Part model, mm, in its own coordinate system. A direction names the side the tool comes from. Round coordinates to 2 decimals unless told otherwise and drop trailing zeros. Write each loop counter-clockwise with the first axis right and the second up, starting at its lowest first coordinate (ties: lowest second). Pieces come first, ordered by that corner, then holes.
```python
from build123d import *

# Parameters (mm, degrees)
SKETCH_1_R          = 2.25
EXTRUDE_2_DEPTH     = 20
SKETCH_7_W          = 2.4
SKETCH_7_H          = 2.4
CUT_EXTRUDE_3_DEPTH = 2.5
SKETCH_9_R          = 3
EXTRUDE_4_DEPTH     = 1
SKETCH_10_W         = 4
SKETCH_10_H         = 4
EXTRUDE_5_DEPTH     = 2
CUT_EXTRUDE_START   = -20
SKETCH_12_OUTSIDE_W = 12.904
SKETCH_12_OUTSIDE_H = 12.904
SKETCH_12_OUTSIDE_R = 1
CUT_EXTRUDE_4_DEPTH = 16.5
FILLET_1_R          = 2


with BuildPart() as part:
    # 草图1 → 凸台-拉伸2 (new body)
    with BuildSketch(Plane.XY):
        Circle(SKETCH_1_R)
    extrude(amount=EXTRUDE_2_DEPTH)

    # 草图7 → 切除-拉伸3 (cut)
    with BuildSketch(Plane.XY):
        Rectangle(SKETCH_7_W, SKETCH_7_H)
    extrude(amount=CUT_EXTRUDE_3_DEPTH, mode=Mode.SUBTRACT)

    # 草图9 → 凸台-拉伸4 (add)
    with BuildSketch(Plane.XY.offset(20)):
        Circle(SKETCH_9_R)
    extrude(amount=EXTRUDE_4_DEPTH)

    # 草图10 → 凸台-拉伸5 (add)
    with BuildSketch(Plane.XY.offset(21)):
        Rectangle(SKETCH_10_W, SKETCH_10_H)
    extrude(amount=EXTRUDE_5_DEPTH)

    # 草图12 outside → 切除-拉伸4 (cut)
    with BuildSketch(Plane(origin=(0, 0, 0), x_dir=(-1, 0, 0), z_dir=(0, 0, -1)).offset(CUT_EXTRUDE_START)):
        Rectangle(SKETCH_12_OUTSIDE_W, SKETCH_12_OUTSIDE_H)
        with Locations(Location((0, 0, 0), (0, 0, 180))):
            Circle(SKETCH_12_OUTSIDE_R, mode=Mode.SUBTRACT)
    extrude(amount=CUT_EXTRUDE_4_DEPTH, mode=Mode.SUBTRACT)

    # 圆角1
    # the kernel refuses this fillet: 2 mm, written as the material it adds along each edge
    with BuildSketch(Plane(origin=(0, 0, 3.5), x_dir=(1, 0, 0), z_dir=(0, 1, 0))) as fillet_1_piece_1:
        with BuildLine():
            CenterArc((3, -1.854049622), FILLET_1_R, 112.024312837, 67.975687163)
            Line((2.25, 0), (2.235, 0.037080992))
            ThreePointArc((2.235, 0.037080992), (1.625, 0.04), (1, 0.04))
            Line((1, 0.04), (0.96, 0))
            Line((0.96, 0), (0.96, -1.854049622))
            Line((0.96, -1.854049622), (1, -1.854049622))
        make_face()
    revolve(axis=Axis((0, 0, 3.5), (0, 0, -1)))
    with BuildSketch(Plane(origin=(0, 0, 20), x_dir=(1, 0, 0), z_dir=(0, 1, 0))) as fillet_1_piece_2:
        with BuildLine():
            CenterArc((1 + FILLET_1_R, FILLET_1_R), FILLET_1_R, 180, 90)
            Line((1, FILLET_1_R), (1 - FILLET_1_R * 0.02, FILLET_1_R))
            Line((1 - FILLET_1_R * 0.02, FILLET_1_R), (1 - FILLET_1_R * 0.02, -FILLET_1_R * 0.02))
            Line((1 - FILLET_1_R * 0.02, -FILLET_1_R * 0.02), (1 + FILLET_1_R, -FILLET_1_R * 0.02))
            Line((1 + FILLET_1_R, -FILLET_1_R * 0.02), (1 + FILLET_1_R, 0))
        make_face()
    revolve(axis=Axis((0, 0, 20), (0, 0, -1)))


solid = part.part
```
Q1. Cut at D-D on z = 6.25. Write the cut outline in (x, y).
Values follow:
outline: circle Ø2 at (0, 0)
Q2. Wall check: L1, parallel to Y at x = -1.05, z = 21.5; L2, parallel to X at y = -1, z = 1.75; L3, parallel to Z at x = 1.7, y = -0.4. Give the ranges that are in metal, low to high.
Values follow:
L1: y = -2 to 2
L2: x = -2.02 to -1.2, 1.2 to 2.02
L3: z = 0 to 3.8, 19.56 to 23
Q3. Which spindle directions (+Z, -Z, +X, -X, +Y, -Y) get a long thin tool onto all of the face, cutting with end or side? Do faces 1 (the flat face through (0, -2, 22)), 2 (the cylindrical face through (-3, 0.1, 20.5)), 3 (the flat face through (0, 0, 2.5)), 4 (the flat face through (-2, 0, 22)), 5 (the flat face through (0, 2, 22)). Say none if no direction does.
Values follow:
face 1: +Z, +X, -X, -Y
face 2: +Z, -Z
face 3: -Z
face 4: +Z, -X, +Y, -Y
face 5: +Z, +X, -X, +Y
Q4. Drop flat-ended pins along their axis: pin 1 (1.2 mm diameter, centred on x = 0, z = 1, fed in from +Y); pin 2 (2 mm diameter, centred on x = -1, z = 22.5, fed in from +Y); pin 3 (1.9 mm diameter, centred on x = 0, z = 1, fed in from -Y). Give the stop position or say it passes through.
Values follow:
pin 1: stops at y = 2.25
pin 2: stops at y = 2
pin 3: stops at y = -2.25
Q5. Cut at C-C on z = 20.25. Write the cut outline in (x, y), plus the area to 3 significant figures.
Values follow:
outline: circle Ø6 at (0, 0)
area: 28.3 mm2
Q6. Cut at A-A on y = 0. Write the cut outline in (x, z).
Values follow:
outline: (-3, 20) arc R2 cw to (-1, 18) - (-1, 5.35) arc R2 cw to (-2.25, 3.5) - (-2.25, 0) - (-1.2, 0) - (-1.2, 2.5) - (1.2, 2.5) - (1.2, 0) - (2.25, 0) - (2.25, 3.5) arc R2 cw to (1, 5.35) - (1, 18) arc R2 cw to (3, 20) - (3, 21) - (2, 21) - (2, 23) - (-2, 23) - (-2, 21) - (-3, 21) - close
Q7. Mould opens along X. For faces 6 (the flat face through (1.2, 0, 1)), 7 (the flat face through (2, 0, 22)), 8 (the cylindrical face through (0, 1, 12)) say: +X half, -X half, draft (parallel to the pull), parting line (faces both ways), or undercut.
Values follow:
face 6: undercut
face 7: +X half
face 8: parting line
